Autodesk Fusion 360 part; units mm, degrees
sketch "스케치1" plane through (0, 0, 0) normal (0, 0, 1) x (1, 0, 0)
  line L0 (0, 0) -> (103, 0)
  line L1 (103, 0) -> (103, 103)
  line L2 (103, 103) -> (0, 103)
  line L3 (0, 103) -> (0, 0)
  line L4 (0, 80.7838) -> (1.5, 80.7838)
  line L5 (4.5156, 103) -> (4.5156, 101.5)
  line L6 (1.5, 101.5) -> (101.5, 101.5)
  line L7 (101.5, 101.5) -> (101.5, 1.5)
  line L8 (101.5, 1.5) -> (1.5, 1.5)
  line L9 (1.5, 1.5) -> (1.5, 101.5)
  line L10 (1.5, 101.5) -> (9.5, 101.5)
  line L11 (9.5, 101.5) -> (9.5, 93.5)
  line L12 (9.5, 93.5) -> (1.5, 93.5)
  line L13 (1.5, 93.5) -> (1.5, 101.5)
  line L14 (1.5, 1.5) -> (9.5, 1.5)
  line L15 (9.5, 1.5) -> (9.5, 9.5)
  line L16 (9.5, 9.5) -> (1.5, 9.5)
  line L17 (1.5, 9.5) -> (1.5, 1.5)
  line L18 (101.5, 1.5) -> (93.5, 1.5)
  line L19 (93.5, 1.5) -> (93.5, 9.5)
  line L20 (93.5, 9.5) -> (101.5, 9.5)
  line L21 (101.5, 9.5) -> (101.5, 1.5)
  line L22 (101.5, 101.5) -> (93.5, 101.5)
  line L23 (93.5, 101.5) -> (93.5, 93.5)
  line L24 (93.5, 93.5) -> (101.5, 93.5)
  line L25 (101.5, 93.5) -> (101.5, 101.5)
  circle A0 centre (5.5, 97.5) radius 1.5
  circle A1 centre (97.5, 97.5) radius 1.4
  circle A2 centre (5.5, 5.5) radius 1.4
  circle A3 centre (97.5, 5.5) radius 1.5
  dimension "d1" = 103
  dimension "d5" = 100
  dimension "d6" = 100
  dimension "d7" = 1.5
  dimension "d8" = 1.5
  dimension "d9" = 1.5
  dimension "d10" = 8
  dimension "d11" = 8
  dimension "d12" = 8
  dimension "d13" = 8
  dimension "d14" = 8
  dimension "d15" = 8
  dimension "d16" = 8
  dimension "d17" = 8
  dimension "d18" = 3
  dimension "d20" = 4
  dimension "d21" = 4
  dimension "d22" = 2.8
  dimension "d23" = 4
  dimension "d24" = 4
  dimension "d25" = 2.8
  dimension "d26" = 4
  dimension "d27" = 4
  dimension "d28" = 3
  dimension "d29" = 4
  dimension "d30" = 4
extrude "돌출1" add sketch "스케치1" along normal blind 5 contours L0 L1 L2 L3 L4 L5 L6 L7 L8 L9 L10 L14 L17 L18 L21 L22 L25 | L2 L3 L4 L5 L6 L9 L10 L13
extrude "돌출2" add sketch "스케치1" along normal blind 3.3 contours L8 L9 L14 L15 L16 L17 | L6 L9 L10 L11 L12 L13 | L6 L7 L22 L23 L24 L25 | L7 L8 L18 L19 L20 L21
extrude "돌출3" add sketch "스케치1" along normal blind 1 contours L6 L7 L8 L9 L11 L12 L15 L16 L19 L20 L23 L24
extrude "돌출4" add sketch "스케치1" along normal blind 1 contours A0 | A1 | A2 | A3
The listing builds one solid part. Answer for the finished solid, in the listing's coordinates (mm). A direction names the side the tool comes from. Round coordinates to 2 decimals unless told otherwise and drop trailing zeros. Write each loop counter-clockwise with the first axis right and the second up, starting at its lowest first coordinate (ties: lowest second). Pieces come first, ordered by that corner, then holes. Notation, with made-up numbers: M -5.5,33 L 1.5,33 A23 cw 1.5,68 Z; hole C 89,-8.75 d4. An arc over 180 degrees is marked long. Write each question's results on one line, items separated by ' | '. Start each with the question number.
Item 1: A cutting plane is placed at B-B on z = 4.1. Write down the section's boundary in (x, y), and give its area (3 significant figures).
Item 2: A cutting plane is placed at C-C on x = 42. Write down the section's boundary in (y, z), and give its area (3 significant figures).
Item 3: Straight lines are drawn through the part: L1, parallel to X at y = 97.5, z = 2.5; L2, parallel to Y at x = 31.5, z = 4. For each, find the intervals that lie inside material, in ascending order. Write a range as [from, to].
Item 4: For a pull along X with two mould halves and no side action, classify faces 1 (the face through (52, 103, 2)), 2 (the face through (0, 52, 2)), 3 (the face through (6, 9.5, 2)) as pulls with the +X half, pulls with the -X half, needs draft (parallel to the pull), parting line crosses it, or undercut.
Item 5: A cutting plane is placed at A-A on y = 5.5. Write down the section's boundary in (x, z).
Item 6: For faces 4 (the face through (51, 0, 2)), 5 (the face through (97, 98, 1)), determine the directions among +Z, -Z, +X, -X, +Y, -Y from which every point of the face is accessible in a straight line to the end or side of a thin tool.
Item 7: Flat-ended cylindrical pins translate along their axes: pin 1 Ø0.9 at (x, y) = (98, 5.5) entering from +Z; pin 2 Ø2 at (x, y) = (98, 97.5) entering from +Z. Find the tip coordinate at first contact, or state that the pin passes through.
Check sheet entries:
1) outline: M 0,0 L 103,0 L 103,103 L 0,103 Z; hole M 1.5,1.5 L 101.5,1.5 L 101.5,101.5 L 1.5,101.5 Z | area: 609 mm²
2) outline: M 0,0 L 103,0 L 103,5 L 101.5,5 L 101.5,1 L 1.5,1 L 1.5,5 L 0,5 Z | area: 115 mm²
3) L1: [0, 4], [7, 9.5], [93.5, 96.1], [98.9, 103] | L2: [0, 1.5], [101.5, 103]
4) face 1: needs draft | face 2: pulls with the -X half | face 3: undercut
5) outline: M 0,0 L 103,0 L 103,5 L 101.5,5 L 101.5,3.3 L 99,3.3 L 99,1 L 96,1 L 96,3.3 L 93.5,3.3 L 93.5,1 L 9.5,1 L 9.5,3.3 L 6.9,3.3 L 6.9,1 L 4.1,1 L 4.1,3.3 L 1.5,3.3 L 1.5,5 L 0,5 Z
6) face 4: +Z, -Z, +X, -X, -Y | face 5: +Z
7) pin 1: z = 1 | pin 2: z = 3.3
